Check sheet for the modelled part. Datum: model origin and axes. Units: mm. Face numbers are marked on the shaded views. A direction names the side the tool comes from. Round coordinates to 2 decimals unless told otherwise and drop trailing zeros. Loops run counter-clockwise (first coordinate to the right, second up) from the corner with the lowest first, then second, coordinate; pieces in that order, holes last. Notation, with made-up numbers: M 44,9 L 99,9 A23 ccw 99,39 Z; hole C 50.25,15.5 d9. An arc over 180 degrees is marked long. One line per question, with ' | ' between items. Start each with the question number.
(1) Thickness scan on probe 1 along X at (y, z) = (149.5, -7); probe 2 along Z at (x, y) = (9, 245.5); probe 3 along Z at (x, y) = (29, 64). Record the ranges inside material, lowest first. Write a range as [from, to].
(2) Section check B-B (y = 244.5). Record the boundary of the cut face in (x, z).
(3) Section check A-A (y = 511). Record the boundary of the cut face in (x, z).
(4) Tool access check on the marked faces 1 and 2. Record the directions out of +Z, -Z, +X, -X, +Y, -Y that give a thin tool (end or side, any length) a straight path to the whole face; none if there is none.
(5) Draft check along Z on the marked faces 3, 4 and 5. Enter one of: +Z half, -Z half, draft (parallel to the pull), parting line (faces both ways), or undercut.
(6) Go/stop test with flat-tipped pins: P1, Ø11, axis at x = 35.5, z = -27, coming from the +Y side; P2, Ø1.6, axis at y = 563.5, z = -0.5, coming from the -X side; P3, Ø1.2, axis at y = 55.5, z = -39.5, coming from the +X side. Record where each tip stops, or that it passes through.
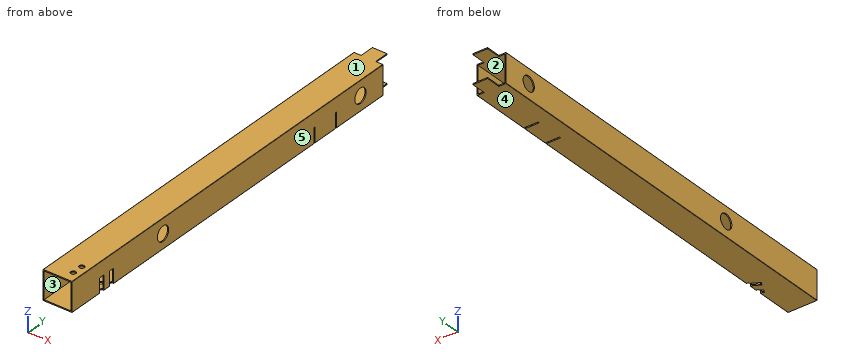
```python
from build123d import *

# Parameters (mm, degrees)
SKETCH1_W           = 37
SKETCH1_H           = 37
BOSS_EXTRUDE1_DEPTH = 571
SKETCH2_W           = 10
SKETCH2_H           = 20
CUT_EXTRUDE1_DEPTH  = 40
SKETCH3_W           = 21
SKETCH3_H           = 2
CUT_EXTRUDE2_DEPTH  = 20
CUT_EXTRUDE3_DEPTH  = 20
SKETCH5_R           = 3.5
CUT_EXTRUDE4_DEPTH  = 10
SKETCH6_R           = 10
CUT_EXTRUDE5_DEPTH  = 574.795259653


with BuildPart() as part:
    # Sketch1 → Boss-Extrude1 (new body)
    with BuildSketch(Plane(origin=(0, 0, 0), x_dir=(1, 0, 0), z_dir=(0, 1, 0))):
        with BuildLine():
            Line((0.5, 0), (39.5, 0))
            ThreePointArc((39.5, 0), (39.853553391, 0.146446609), (40, 0.5))
            Line((40, 0.5), (40, 39.5))
            ThreePointArc((40, 39.5), (39.853553391, 39.853553391), (39.5, 40))
            Line((39.5, 40), (0.5, 40))
            ThreePointArc((0.5, 40), (0.146446609, 39.853553391), (0, 39.5))
            Line((0, 39.5), (0, 0.5))
            ThreePointArc((0, 0.5), (0.146446609, 0.146446609), (0.5, 0))
        make_face()
        with Locations((20, 20)):
            Rectangle(SKETCH1_W, SKETCH1_H, mode=Mode.SUBTRACT)
    extrude(amount=BOSS_EXTRUDE1_DEPTH)

    # Sketch2 → Cut-Extrude1 (cut)
    with BuildSketch(Plane.XY.offset(-40)):
        with Locations((35, 561)):
            Rectangle(SKETCH2_W, SKETCH2_H)
        with Locations((5, 561)):
            Rectangle(SKETCH2_W, SKETCH2_H)
    extrude(amount=CUT_EXTRUDE1_DEPTH, mode=Mode.SUBTRACT)

    # Sketch3 → Cut-Extrude2 (cut)
    with BuildSketch(Plane(origin=(40, 0, 0), x_dir=(0, 0, -1), z_dir=(1, 0, 0))):
        with Locations((29.5, 467.5)):
            Rectangle(SKETCH3_W, SKETCH3_H)
        with Locations((29.5, 429.5)):
            Rectangle(SKETCH3_W, SKETCH3_H)
    extrude(amount=-CUT_EXTRUDE2_DEPTH, mode=Mode.SUBTRACT)

    # Sketch4 → Cut-Extrude3 (cut)
    with BuildSketch(Plane(origin=(0, 0, -40), x_dir=(-1, 0, 0), z_dir=(0, 0, -1))):
        Polygon((-40, 73.59987752), (-37, 73.59987752), (-37, 71.867826713), (-25.659711467, 65.320508076), (-28.159711467, 60.990381057), (-37, 66.094324021), (-40, 66.094324021), align=None)
        Polygon((-40, 56.279369445), (-37, 56.279369445), (-37, 54.547318637), (-32.726698765, 52.080127019), (-35.226698765, 47.75), (-37, 48.773815945), (-40, 48.773815945), align=None)
    extrude(amount=-CUT_EXTRUDE3_DEPTH, mode=Mode.SUBTRACT)

    # Sketch5 → Cut-Extrude4 (cut)
    with BuildSketch(Plane.XY):
        with Locations((30, 15)):
            Circle(SKETCH5_R)
        with Locations((30, 30)):
            Circle(SKETCH5_R)
    extrude(amount=-CUT_EXTRUDE4_DEPTH, mode=Mode.SUBTRACT)

    # Sketch6 → Cut-Extrude5 (cut, through all)
    with BuildSketch(Plane.ZY):
        with Locations((-20, 511)):
            Circle(SKETCH6_R)
        with Locations((-20, 161)):
            Circle(SKETCH6_R)
    extrude(amount=-CUT_EXTRUDE5_DEPTH, mode=Mode.SUBTRACT)


solid = part.part
```
The answers:
1) probe 1: [0, 1.5], [38.5, 40] | probe 2: [-40, -38.5], [-1.5, 0] | probe 3: [-1.5, 0]
2) outline: M 0,-39.5 A0.5 ccw 0.5,-40 L 39.5,-40 A0.5 ccw 40,-39.5 L 40,-0.5 A0.5 ccw 39.5,0 L 0.5,0 A0.5 ccw 0,-0.5 Z; hole M 1.5,-38.5 L 38.5,-38.5 L 38.5,-1.5 L 1.5,-1.5 Z
3) outline: M 0,-39.5 A0.5 ccw 0.5,-40 L 39.5,-40 A0.5 ccw 40,-39.5 L 40,-30 L 38.5,-30 L 38.5,-38.5 L 1.5,-38.5 L 1.5,-30 L 0,-30 Z; M 0,-10 L 1.5,-10 L 1.5,-1.5 L 38.5,-1.5 L 38.5,-10 L 40,-10 L 40,-0.5 A0.5 ccw 39.5,0 L 0.5,0 A0.5 ccw 0,-0.5 Z
4) face 1: +Z, +X, -X, +Y, -Y | face 2: +Y, -Y
5) face 3: undercut | face 4: -Z half | face 5: draft
6) P1: y = 551 | P2: x = 10 | P3: x = 37
